Job drawing, mm, ordinate dimensions from the low corner. One solid piece. A direction names the side the tool comes from. Round coordinates to 2 decimals unless told otherwise and drop trailing zeros. Loops run counter-clockwise (first coordinate to the right, second up) from the corner with the lowest first, then second, coordinate; pieces in that order, holes last.
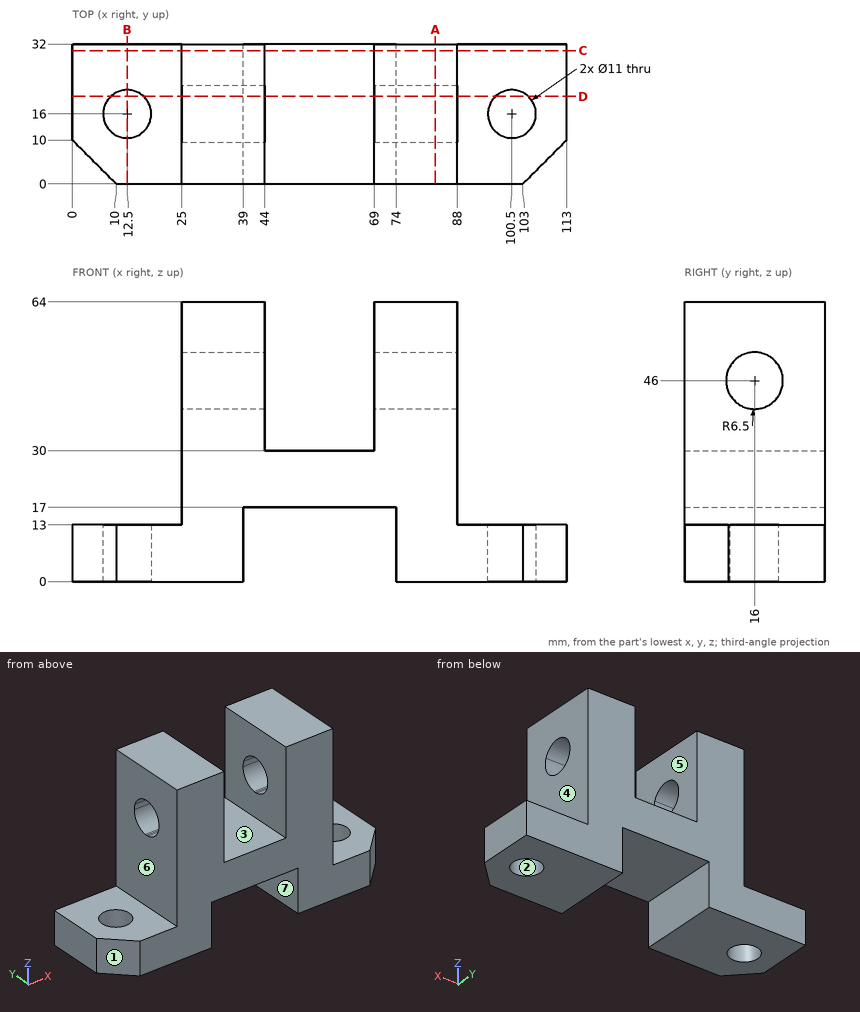
Item 1: 3-axis set-ups, long thin cutter, end or side, ignore diameter. For the marked faces 4, 5, 6 and 7: which of +Z, -Z, +X, -X, +Y, -Y reach the whole face in a straight line?
Answers follow:
face 4: +Z, +X, +Y, -Y
face 5: +Z, +Y, -Y
face 6: +Z, -X, +Y, -Y
face 7: -Z, +Y, -Y
Item 2: Cut at B-B, the plane x = 12.5. Give the cut face in (y, z).
Answers follow:
outline: (0, 0) - (10.5, 0) - (10.5, 13) - (0, 13) - close; (21.5, 0) - (32, 0) - (32, 13) - (21.5, 13) - close
Item 3: Cut at A-A, the plane x = 83. Give the cut face in (y, z), plus the area to 3 significant figures.
Answers follow:
outline: (0, 0) - (32, 0) - (32, 64) - (0, 64) - close; hole circle Ø13 at (16, 46)
area: 1,920 mm2
Item 4: Probe line 1 (X direction, y = 3, z = 39); line 2 (X direction, y = 3, z = 14); line 3 (Y direction, x = 100.5, z = 10). List the from-to ranges inside material, lowest first.
Answers follow:
line 1: x = 25 to 44, 69 to 88
line 2: x = 25 to 39, 74 to 88
line 3: y = 0 to 10.5, 21.5 to 32
Item 5: Cut at D-D, the plane y = 20. State how many separate pieces and enclosed holes the cut face has, plus the area to 3 significant figures.
Answers follow:
separate pieces: 5
enclosed holes: 0
area: 2,650 mm2
Item 6: Flat gauge pins, fed straight in: P1, Ø16, axis at y = 18, z = 38.5, coming from the +X side; P2, Ø7.5, axis at x = 18.5, y = 11.5, coming from the +Z side; P3, Ø4, axis at x = 57.5, y = 5, coming from the -Z side. Where does each tip first touch, or does it go through?
Answers follow:
P1: stops at x = 88
P2: stops at z = 13
P3: stops at z = 17
Item 7: Two-plate mould, pull along Y, no slides. Class the marked faces 1, 2 and 3: released by +Y, released by -Y, zero draft, split by the parting line, or undercut.
Answers follow:
face 1: released by -Y
face 2: undercut
face 3: zero draft
Item 8: Cut at C-C, the plane y = 30.5. Give the cut face in (x, z).
Answers follow:
outline: (0, 0) - (39, 0) - (39, 17) - (74, 17) - (74, 0) - (113, 0) - (113, 13) - (88, 13) - (88, 64) - (69, 64) - (69, 30) - (44, 30) - (44, 64) - (25, 64) - (25, 13) - (0, 13) - close
